Check sheet for the modelled part. Datum: model origin and axes. Units: mm. Face numbers are marked on the shaded views. A direction names the side the tool comes from. Give positions to 0.01 mm unless a question says otherwise; leave off trailing zeros. Write each loop counter-clockwise with the first axis right and the second up, starting at its lowest first coordinate (ties: lowest second). Pieces come first, ordered by that corner, then holes. Notation, with made-up numbers: M 59.5,78 L 104.5,78 A18 cw 104.5,98 Z; hole C 0.5,6.25 d10. An arc over 180 degrees is marked long. Write item = value, one per line. Start each with the question number.
1) Mould release check, pull along X, two halves, no side actions. Record for the marked faces 1, 2 and 3: released by +X, released by -X, zero draft, split by the parting line, or undercut.
2) Access from +Z, -Z, +X, -X, +Y, -Y to the whole of each face (thin tool, end or side, straight path). Record for the marked faces 4 and 5.
3) Cross-section at A-A, the plane y = -5. Record the cut outline in (x, z), plus the area to 3 significant figures.
4) Cross-section at B-B, the plane z = 33. Record the cut outline in (x, y), plus the area to 3 significant figures.
5) Scan lines: line 1 along X through (y, z) = (-2.75, -71); line 2 along Y through (x, z) = (11, -71); line 3 along X through (y, z) = (-1.25, -19). Record each from-to range of solid material in increasing order. Write a range as [from, to].
6) Go/stop test with flat-tipped pins: pin 1 (0.6 mm diameter, centred on x = 16, z = -76.5, fed in from +Y); pin 2 (0.6 mm diameter, centred on x = -16, z = 30.5, fed in from -Y); pin 3 (8 mm diameter, centred on x = 4, z = -25, fed in from -Y). Record where each tip stops, or that it passes through.
7) Cross-section at C-C, the plane y = -19.25. Record the cut outline in (x, z).
8) Cross-section at D-D, the plane x = 7.5. Record the cut outline in (y, z).
```python
from build123d import *

# Parameters (mm, degrees)
BOSS_EXTRUDE1_DEPTH = 75
BOSS_EXTRUDE2_DEPTH = 0.25
BOSS_EXTRUDE3_DEPTH = 0.25


with BuildPart() as part:
    # Sketch2 → Boss-Extrude1 (new, symmetric)
    with BuildSketch(Plane.XY):
        with BuildLine():
            Line((15.5, -24), (15.5, -2))
            ThreePointArc((15.5, -2), (14.914213562, -0.585786438), (13.5, 0))
            Line((13.5, 0), (-13.5, 0))
            ThreePointArc((-13.5, 0), (-14.914213562, -0.585786438), (-15.5, -2))
            Line((-15.5, -2), (-15.5, -23))
            Line((-15.5, -23), (-16, -23))
            Line((-16, -23), (-16, -2))
            ThreePointArc((-16, -2), (-15.267766953, -0.232233047), (-13.5, 0.5))
            Line((-13.5, 0.5), (13.5, 0.5))
            ThreePointArc((13.5, 0.5), (15.267766953, -0.232233047), (16, -2))
            Line((16, -2), (16, -24))
            Line((16, -24), (15.5, -24))
        make_face()
    extrude(amount=BOSS_EXTRUDE1_DEPTH, both=True)

    # Sketch3 → Boss-Extrude2 (add, symmetric)
    with BuildSketch(Plane(origin=(15.75, 0, 0), x_dir=(0, 0, -1), z_dir=(1, 0, 0))):
        with BuildLine():
            Line((-75, -24), (-78, -24))
            ThreePointArc((-78, -24), (-78.707106781, -23.707106781), (-79, -23))
            Line((-79, -23), (-79, -17))
            ThreePointArc((-79, -17), (-78.707106781, -16.292893219), (-78, -16))
            Line((-78, -16), (-75, -16))
            Line((-75, -16), (-75, -24))
        make_face()
        with BuildLine():
            Line((75, -24), (78, -24))
            ThreePointArc((78, -24), (78.707106781, -23.707106781), (79, -23))
            Line((79, -23), (79, -17))
            ThreePointArc((79, -17), (78.707106781, -16.292893219), (78, -16))
            Line((78, -16), (75, -16))
            Line((75, -16), (75, -24))
        make_face()
    extrude(amount=BOSS_EXTRUDE2_DEPTH, both=True)

    # Sketch4 → Boss-Extrude3 (add, symmetric)
    with BuildSketch(Plane(origin=(-15.75, 0, 0), x_dir=(0, 0, -1), z_dir=(1, 0, 0))):
        with BuildLine():
            Line((-75, -23), (-78, -23))
            ThreePointArc((-78, -23), (-78.707106781, -22.707106781), (-79, -22))
            Line((-79, -22), (-79, -16))
            ThreePointArc((-79, -16), (-78.707106781, -15.292893219), (-78, -15))
            Line((-78, -15), (-75, -15))
            Line((-75, -15), (-75, -23))
        make_face()
        with BuildLine():
            Line((79, -22), (79, -16))
            ThreePointArc((79, -16), (78.707106781, -15.292893219), (78, -15))
            Line((78, -15), (75, -15))
            Line((75, -15), (75, -23))
            Line((75, -23), (78, -23))
            ThreePointArc((78, -23), (78.707106781, -22.707106781), (79, -22))
        make_face()
    extrude(amount=BOSS_EXTRUDE3_DEPTH, both=True)


solid = part.part
```
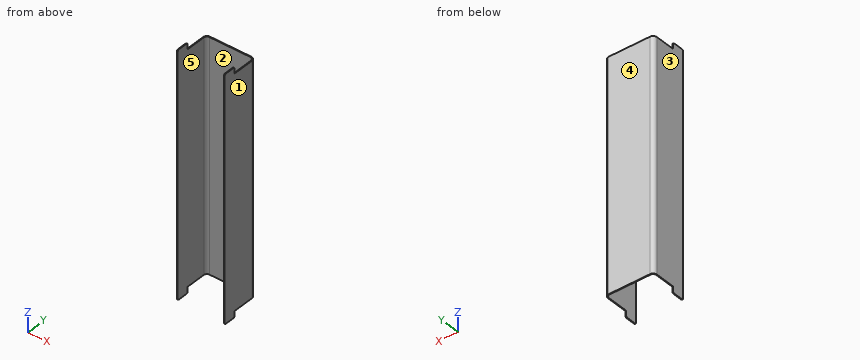
Reply:
q1.face_1 = released by +X
q1.face_2 = undercut
q1.face_3 = released by -X
q2.face_4 = +Z, -Z, +X, -X, +Y
q2.face_5 = +Z, -Z, -Y
q3.outline = M -16,-75 L -15.5,-75 L -15.5,75 L -16,75 Z; M 15.5,-75 L 16,-75 L 16,75 L 15.5,75 Z
q3.area = 150 mm2
q4.outline = M -16,-23 L -15.5,-23 L -15.5,-2 A2 cw -13.5,0 L 13.5,0 A2 cw 15.5,-2 L 15.5,-24 L 16,-24 L 16,-2 A2.5 ccw 13.5,0.5 L -13.5,0.5 A2.5 ccw -16,-2 Z
q4.area = 38.5 mm2
q5.line_1 = [-16, -15.5], [15.5, 16]
q5.line_2 = [0, 0.5]
q5.line_3 = [-15.88, -15.35], [15.35, 15.88]
q6.pin_1 = -16
q6.pin_2 = -23
q6.pin_3 = 0
q7.outline = M -16,-79 L -15.5,-79 L -15.5,79 L -16,79 Z; M 15.5,-79 L 16,-79 L 16,79 L 15.5,79 Z
q8.outline = M 0,-75 L 0.5,-75 L 0.5,75 L 0,75 Z
